Verification items for the finished model (mm, model axes). A direction names the side the tool comes from. Round coordinates to 2 decimals unless told otherwise and drop trailing zeros. Loops run counter-clockwise (first coordinate to the right, second up) from the corner with the lowest first, then second, coordinate; pieces in that order, holes last. Notation, with made-up numbers: (-9.75, 15) - (1.25, 15) arc R26 cw to (1.25, 35) - close; hole circle Ø8 at (5.5, 33.25). An arc over 180 degrees is marked (long way). Use a Markdown table: item, result. Add a question column.
```python
from build123d import *

# Parameters (mm, degrees)
BOSS_EXTRUDE1_DEPTH = 8
CUT_EXTRUDE5_REACH  = 35.361
SKETCH4_W           = 2
SKETCH4_H           = 4
SKETCH5_W           = 21
SKETCH5_H           = 3.6
CUT_EXTRUDE2_DEPTH  = 6.75
SKETCH6_R           = 1.6
CUT_EXTRUDE3_DEPTH  = 8
CUT_EXTRUDE4_DEPTH  = 3
FILLET1_R           = 4


with BuildPart() as part:
    # Sketch2 → Boss-Extrude1 (new body)
    with BuildSketch(Plane(origin=(0, 0, 0), x_dir=(0, 0, -1), z_dir=(1, 0, 0))):
        with BuildLine():
            Line((-3.5, 7.1), (24.5, 7.1))
            ThreePointArc((24.5, 7.1), (31.6, 0), (24.5, -7.1))
            Line((24.5, -7.1), (-3.5, -7.1))
            ThreePointArc((-3.5, -7.1), (-10.6, 0), (-3.5, 7.1))
        make_face()
    extrude(amount=BOSS_EXTRUDE1_DEPTH)

    # Sketch4 → Cut-Extrude5 (cut, up to next)
    with BuildSketch(Plane.XY, mode=Mode.PRIVATE) as cut_extrude5_sk1:
        with Locations((1, 0)):
            Rectangle(SKETCH4_W, SKETCH4_H)
    cut_extrude5_tool1 = extrude(cut_extrude5_sk1.sketch, amount=-CUT_EXTRUDE5_REACH, mode=Mode.PRIVATE) & part.part
    add(cut_extrude5_tool1.solids().sort_by_distance((1, 0, 0))[0], mode=Mode.SUBTRACT)

    # Sketch5 → Cut-Extrude2 (cut)
    with BuildSketch(Plane(origin=(0, 0, 0), x_dir=(0, 0, -1), z_dir=(1, 0, 0))):
        with Locations((10.5, 3.8)):
            Rectangle(SKETCH5_W, SKETCH5_H)
        with Locations((10.5, -3.8)):
            Rectangle(SKETCH5_W, SKETCH5_H)
    extrude(amount=CUT_EXTRUDE2_DEPTH, mode=Mode.SUBTRACT)

    # Sketch6 → Cut-Extrude3 (cut)
    with BuildSketch(Plane(origin=(8, 0, 0), x_dir=(0, 0, -1), z_dir=(1, 0, 0))):
        with Locations((-3.5, 3.8)):
            Circle(SKETCH6_R)
        with Locations((-3.5, -3.8)):
            Circle(SKETCH6_R)
        with Locations((24.5, 3.8)):
            Circle(SKETCH6_R)
        with Locations((24.5, -3.8)):
            Circle(SKETCH6_R)
    extrude(amount=-CUT_EXTRUDE3_DEPTH, mode=Mode.SUBTRACT)

    # Sketch7 → Cut-Extrude4 (cut)
    with BuildSketch(Plane(origin=(8, 0, 0), x_dir=(0, 0, -1), z_dir=(1, 0, 0))):
        Polygon((-0.7, 2.183419246), (-0.7, 5.416580754), (-3.5, 7.033161507), (-6.3, 5.416580754), (-6.3, 2.183419246), (-3.5, 0.566838493), align=None)
        Polygon((21.7, 5.416580754), (21.7, 2.183419246), (24.5, 0.566838493), (27.3, 2.183419246), (27.3, 5.416580754), (24.5, 7.033161507), align=None)
        Polygon((21.7, -2.183419246), (21.7, -5.416580754), (24.5, -7.033161507), (27.3, -5.416580754), (27.3, -2.183419246), (24.5, -0.566838493), align=None)
        Polygon((-3.5, -7.033161507), (-0.7, -5.416580754), (-0.7, -2.183419246), (-3.5, -0.566838493), (-6.3, -2.183419246), (-6.3, -5.416580754), align=None)
    extrude(amount=-CUT_EXTRUDE4_DEPTH, mode=Mode.SUBTRACT)

    # Fillet1
    # the kernel refuses this fillet: 4 mm, written as the material it takes off along each edge
    with BuildSketch(Plane(origin=(8, 7.1, 3.5), x_dir=(0, -1, 0), z_dir=(0, 0, -1))) as fillet1_piece_1:
        with BuildLine():
            CenterArc((FILLET1_R, FILLET1_R), FILLET1_R, 180, 90)
            Line((0, FILLET1_R), (0, 0))
            Line((0, 0), (FILLET1_R, 0))
        make_face()
    extrude(amount=28, mode=Mode.SUBTRACT)
    with BuildSketch(Plane(origin=(8, 0, -24.5), x_dir=(0, 1, 0), z_dir=(0, 0, 1))) as fillet1_piece_2:
        with BuildLine():
            CenterArc((7.1 - FILLET1_R, FILLET1_R), FILLET1_R, 270, 90)
            Line((7.1 - FILLET1_R, 0), (7.1, 0))
            Line((7.1, 0), (7.1, FILLET1_R))
        make_face()
    revolve(axis=Axis((8, 0, -24.5), (-1, 0, 0)), revolution_arc=180, mode=Mode.SUBTRACT)
    with BuildSketch(Plane(origin=(8, -7.1, -24.5), x_dir=(-1, 0, 0), z_dir=(0, 0, 1))) as fillet1_piece_3:
        with BuildLine():
            CenterArc((FILLET1_R, -FILLET1_R), FILLET1_R, 90, 90)
            Line((0, -FILLET1_R), (0, 0))
            Line((0, 0), (FILLET1_R, 0))
        make_face()
    extrude(amount=28, mode=Mode.SUBTRACT)
    with BuildSketch(Plane(origin=(8, 0, 3.5), x_dir=(0, -1, 0), z_dir=(0, 0, -1))) as fillet1_piece_4:
        with BuildLine():
            CenterArc((7.1 - FILLET1_R, FILLET1_R), FILLET1_R, 270, 90)
            Line((7.1, FILLET1_R), (7.1, 0))
            Line((7.1, 0), (7.1 - FILLET1_R, 0))
        make_face()
    revolve(axis=Axis((8, 0, 3.5), (-1, 0, 0)), revolution_arc=180, mode=Mode.SUBTRACT)


solid = part.part
```
Q1. Go/stop test with flat-tipped pins: pin 1 Ø3 at (y, z) = (-4, -14) entering from -X; pin 2 Ø1 at (x, y) = (3, -3) entering from +Z; pin 3 Ø3.5 at (x, y) = (7, 3) entering from -Z; pin 4 Ø1.9 at (y, z) = (3.8, -24.5) entering from +X. Record where each tip stops, or that it passes through.
Q2. Set-up check for faces 1 (the face through (1.8, -0.1, 0)), 2 (the face through (5.895, 6.033, -22.767)), 3 (the face through (1, 2, -26)): record each of +Z, -Z, +X, -X, +Y, -Y from which the full face is reachable in a straight line by a thin tool's end or side.
Q3. Section check A-A on x = 0.5. Record the cut outline in (y, z), plus the area to 3 significant figures.
Q4. Thickness scan on line 1 along Y through (x, z) = (1.65, -24.5); line 2 along Y through (x, z) = (1.05, 3.5); line 3 along Y through (x, z) = (5.5, -9.5). Record the ranges inside material, lowest first.
Q5. Section check B-B on z = -0.5. Record the cut outline in (x, y).
Q6. Section check C-C on y = -3.8. State how many separate pieces and enclosed holes the cut face has, plus the area to 3 significant figures.
Determined:
| question | item | result |
|---|---|---|
| 1 | pin 1 | stops at x = 6.75 |
| 1 | pin 2 | stops at z = 10.15 |
| 1 | pin 3 | stops at z = -30.98 |
| 1 | pin 4 | passes through |
| 2 | face 1 | -X |
| 2 | face 2 | +X |
| 2 | face 3 | -Z, -X |
| 3 | outline | (-7.1, -24.5) arc R7.1 ccw to (-2, -31.31) - (-2, -21) - (-5.6, -21) - (-5.6, 0) - (5.6, 0) - (5.6, -21) - (2, -21) - (2, -31.31) arc R7.1 ccw to (7.1, -24.5) - (7.1, 3.5) arc R7.1 ccw to (-7.1, 3.5) - close; hole circle Ø3.2 at (-3.8, -24.5); hole circle Ø3.2 at (-3.8, 3.5); hole circle Ø3.2 at (3.8, -24.5); hole circle Ø3.2 at (3.8, 3.5) |
| 3 | area | 247 mm² |
| 4 | line 1 | y = -7.1 to -5.4, -2.2 to -2, 2 to 2.2, 5.4 to 7.1 |
| 4 | line 2 | y = -7.1 to -5.4, -2.2 to 2.2, 5.4 to 7.1 |
| 4 | line 3 | y = -6.81 to -5.6, -2 to 2, 5.6 to 6.81 |
| 5 | outline | (0, -7.1) - (4, -7.1) arc R4 ccw to (8, -3.1) - (8, 3.1) arc R4 ccw to (4, 7.1) - (0, 7.1) - (0, 5.6) - (6.75, 5.6) - (6.75, 2) - (2, 2) - (2, -2) - (6.75, -2) - (6.75, -5.6) - (0, -5.6) - close |
| 6 | separate pieces | 3 |
| 6 | enclosed holes | 0 |
| 6 | area | 103 mm² |
